Work out the finished part from the listing and answer in its coordinate system (mm). A direction names the side the tool comes from. Give positions to 0.01 mm unless a question says otherwise; leave off trailing zeros. Order: outer loops, then holes, each group sorted by start corner. A loop starts at its lowest first (then second) coordinate and runs counter-clockwise, first axis right, second up. Notation, with made-up numbers: M -36,1 L 13,1 A34 ccw 13,40 Z; hole C 56,2.25 d9. An arc over 180 degrees is marked long. One line per item, written item: value.
from build123d import *

# Parameters (mm, degrees)
SKETCH2_R           = 1.5
BOSS_EXTRUDE1_DEPTH = 5
SKETCH4_R           = 1.5
CUT_EXTRUDE1_DEPTH  = 51.652969899


with BuildPart() as part:
    # Sketch2 → Boss-Extrude1 (new body)
    with BuildSketch(Plane(origin=(0, 0, 0), x_dir=(1, 0, 0), z_dir=(0, 1, 0))):
        Polygon((-70.88750853, 28.608973411), (-23.38750853, 28.608973411), (-23.38750853, 19.608973411), (-29.38750853, 19.608973411), (-29.38750853, 13.608973411), (-64.88750853, 13.608973411), (-64.88750853, 19.608973411), (-70.88750853, 19.608973411), align=None)
        with Locations(Location((-60.88750853, 24.518639814, 0), (0, 0, 270))):
            Circle(SKETCH2_R, mode=Mode.SUBTRACT)
        with Locations(Location((-33.38750853, 24.518639814, 0), (0, 0, 270))):
            Circle(SKETCH2_R, mode=Mode.SUBTRACT)
    extrude(amount=BOSS_EXTRUDE1_DEPTH)

    # Sketch4 → Cut-Extrude1 (cut, through all)
    with BuildSketch(Plane.ZY.offset(64.88750853)):
        with Locations((-15.608973411, 2.5)):
            Circle(SKETCH4_R)
    extrude(amount=-CUT_EXTRUDE1_DEPTH, mode=Mode.SUBTRACT)


solid = part.part
(1) Given P1, Ø2.5, axis at x = -26, y = 2.5, coming from the +Z side; P2, Ø2.5, axis at y = 3, z = -17.5, coming from the -X side, each flat-ended and moving along its own axis, determine where each tip first touches the part or whether it passes through.
Findings:
P1: stops at z = -19.61
P2: stops at x = -64.89
(2) Section B-B, the plane x = -60 is taken. Give the vertices of the cut face in (y, z).
Findings:
outline: M 0,-28.61 L 5,-28.61 L 5,-25.73 L 0,-25.73 Z; M 0,-23.31 L 5,-23.31 L 5,-13.61 L 0,-13.61 Z; hole C 2.5,-15.61 d3
(3) Determine the mould class of faces 1 (the flat face through (-47, 5, -21)), 2 (the flat face through (-47, 2, -28.609)), 3 (the cylindrical face through (-47.39, 1.59, -16.8)) for opening direction Y: pulls with the +Y half, pulls with the -Y half, needs draft (parallel to the pull), parting line crosses it, or undercut.
Findings:
face 1: pulls with the +Y half
face 2: needs draft
face 3: undercut
(4) Section A-A, the plane y = 3.05 is taken. Give the vertices of the cut face in (x, z).
Findings:
outline: M -70.89,-28.61 L -23.39,-28.61 L -23.39,-19.61 L -29.39,-19.61 L -29.39,-17 L -64.89,-17 L -64.89,-19.61 L -70.89,-19.61 Z; M -64.89,-14.21 L -29.39,-14.21 L -29.39,-13.61 L -64.89,-13.61 Z; hole C -60.89,-24.52 d3; hole C -33.39,-24.52 d3
(5) Which of the six approach directions +Z, -Z, +X, -X, +Y, -Y give full straight-line access (tool end or side, diameter ignored) to faces 4 (the flat face through (-68, 2, -19.609)), 5 (the flat face through (-47, 2, -13.609)), 6 (the flat face through (-26, 2, -19.609))?
Findings:
face 4: +Z, -X, +Y, -Y
face 5: +Z, +X, -X, +Y, -Y
face 6: +Z, +X, +Y, -Y
(6) Section C-C, the plane z = -23.75 is taken. Give the vertices of the cut face in (x, y).
Findings:
outline: M -70.89,0 L -62.18,0 L -62.18,5 L -70.89,5 Z; M -59.6,0 L -34.68,0 L -34.68,5 L -59.6,5 Z; M -32.1,0 L -23.39,0 L -23.39,5 L -32.1,5 Z
(7) Section D-D, the plane x = -54 is taken. Give the vertices of the cut face in (y, z).
Findings:
outline: M 0,-28.61 L 5,-28.61 L 5,-13.61 L 0,-13.61 Z; hole C 2.5,-15.61 d3
(8) Find the intervals of material crossed by probe 1 along X at (y, z) = (1.5, -24.5); probe 2 along Z at (x, y) = (-31, 2.35); probe 3 along X at (y, z) = (1.9, -25.75), in increasing order. Write a range as from..to.
Findings:
probe 1: x = -70.89..-62.39, -59.39..-34.89, -31.89..-23.39
probe 2: z = -28.61..-17.1, -14.12..-13.61
probe 3: x = -70.89..-61.74, -60.03..-34.24, -32.53..-23.39
